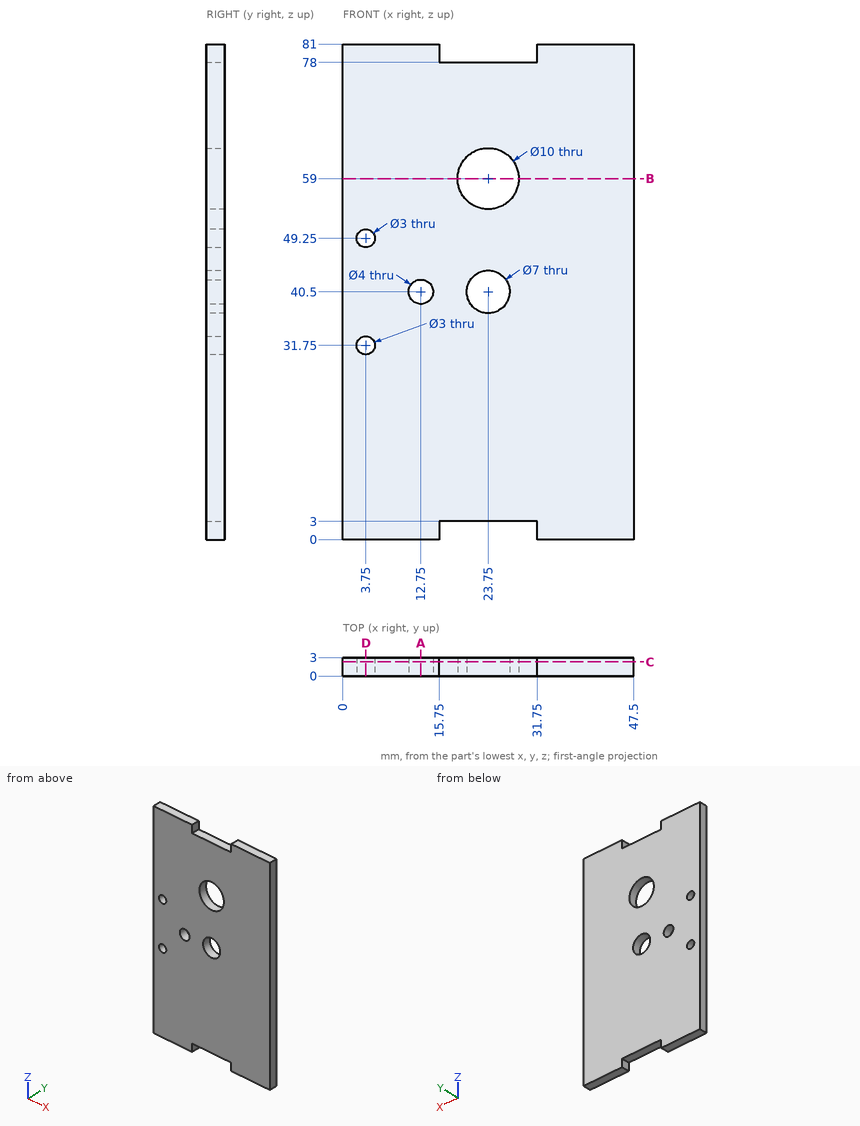
Source: three-view drawing plus pictorial views. Frame: mm from the lowest corner of the part. Round coordinates to 2 decimals unless told otherwise and drop trailing zeros. Order: outer loops, then holes, each group sorted by start corner. A loop starts at its lowest first (then second) coordinate and runs counter-clockwise, first axis right, second up. Notation, with made-up numbers: (13, -26) - (41, -26) arc R15 ccw to (41, -17) - close; hole circle Ø2 at (30, 61). An arc over 180 degrees is marked (long way). Answer in a Markdown table with one row per item.
Item 1: Section query D-D (x = 3.75). Return the cut outline in (y, z).
Model answer:
| item | result |
|---|---|
| outline | (0, 0) - (3, 0) - (3, 30.25) - (0, 30.25) - close; (0, 33.25) - (3, 33.25) - (3, 47.75) - (0, 47.75) - close; (0, 50.75) - (3, 50.75) - (3, 81) - (0, 81) - close |
Item 2: Section query B-B (z = 59). Return the cut outline in (x, y).
Model answer:
| item | result |
|---|---|
| outline | (0, 0) - (18.75, 0) - (18.75, 3) - (0, 3) - close; (28.75, 0) - (47.5, 0) - (47.5, 3) - (28.75, 3) - close |
Item 3: Pin query (flat end, axial travel): pin 1 (1 mm diameter, centred on x = 26, z = 72.5, fed in from -Y); pin 2 (1.5 mm diameter, centred on x = 27, y = 2, fed in from +Z). Return the tip coordinate at first contact, or that it passes through.
Model answer:
| item | result |
|---|---|
| pin 1 | stops at y = 0 |
| pin 2 | stops at z = 78 |
Item 4: Section query A-A (x = 12.75). Return the cut outline in (y, z), then the cut area to 3 significant figures.
Model answer:
| item | result |
|---|---|
| outline | (0, 0) - (3, 0) - (3, 38.5) - (0, 38.5) - close; (0, 42.5) - (3, 42.5) - (3, 81) - (0, 81) - close |
| area | 231 mm² |
Item 5: Section query C-C (y = 2.3). Return the cut outline in (x, z).
Model answer:
| item | result |
|---|---|
| outline | (0, 0) - (15.75, 0) - (15.75, 3) - (31.75, 3) - (31.75, 0) - (47.5, 0) - (47.5, 81) - (31.75, 81) - (31.75, 78) - (15.75, 78) - (15.75, 81) - (0, 81) - close; hole circle Ø3 at (3.75, 31.75); hole circle Ø3 at (3.75, 49.25); hole circle Ø4 at (12.75, 40.5); hole circle Ø10 at (23.75, 59); hole circle Ø7 at (23.75, 40.5) |
Item 6: Line query: line 1 (X direction, y = 1.45, z = 40.5); line 2 (X direction, y = 1.15, z = 31.75); line 3 (Z direction, x = 21, y = 1.35). Output: solid intervals per line, ascending.
Model answer:
| item | result |
|---|---|
| line 1 | x = 0 to 10.75, 14.75 to 20.25, 27.25 to 47.5 |
| line 2 | x = 0 to 2.25, 5.25 to 47.5 |
| line 3 | z = 3 to 38.33, 42.67 to 54.82, 63.18 to 78 |
